For this review, take the finished solid that the model builds, in its own axes (mm). A direction names the side the tool comes from. Coordinates: 2 decimals unless noted, no trailing zeros. Order: outer loops, then holes, each group sorted by start corner. A loop starts at its lowest first (then second) coordinate and runs counter-clockwise, first axis right, second up. Notation, with made-up numbers: (29.5, 30) - (39.5, 30) arc R25 ccw to (39.5, 52) - close; hole circle Ø3 at (80.25, 0.5). An arc over 180 degrees is marked (long way). One line per item, written item: value. Start each with the question number.
(1) For faces 1 (the flat face through (238, 0, -1)), 2 (the flat face through (-3, 5, -50)), list the 3-axis set-ups (+Z, -Z, +X, -X, +Y, -Y) from which the entire face can be reached by the end or side of a thin tool; tool diameter is ignored.
(2) Clearance check with flat-ended pins moving along their axes: pin 1 (11 mm diameter, centred on x = 81.5, y = 6.5, fed in from -Z); pin 2 (5 mm diameter, centred on x = -92.5, z = -55.5, fed in from +Y). State where each tip first meets the part, or that it passes through.
(3) Consider section B-B on y = 4.25. Write out the cut boundary in (x, z), then the cut area to 3 significant figures.
(4) To check wall thickness, follow line 1 along Z through (x, y) = (-135, 6.5); line 2 along Y through (x, z) = (-32, -53.5). State the ranges of each line that lie inside material, in increasing order.
(5) Consider section A-A on x = -72.5. Write out the cut boundary in (y, z), then the cut area to 3 significant figures.
```python
from build123d import *

# Parameters (mm, degrees)
F0_W     = 476
F0_H     = 10
F1_DEPTH = 10
F0_H_2   = 110
F2_DEPTH = 10


with BuildPart() as f1:
    # F0 (on Front) → F1 (new body)
    with BuildSketch(Plane.XZ):
        with Locations((0, -55)):
            Rectangle(F0_W, F0_H)
    extrude(amount=F1_DEPTH)

    # F0 (on Front) → F2 (join, symmetric)
    with BuildSketch(Plane.XZ):
        with Locations((0, 5)):
            Rectangle(F0_W, F0_H_2)
    extrude(amount=F2_DEPTH, both=True)


solid = f1.part
```
Geometry check:
1. face 1: +Z, -Z, +X, +Y, -Y
1. face 2: -Z, +X, -X, +Y
2. pin 1: stops at z = -50
2. pin 2: stops at y = 0
3. outline: (-238, -50) - (238, -50) - (238, 60) - (-238, 60) - close
3. area: 52,400 mm^2
4. line 1: z = -50 to 60
4. line 2: y = -10 to 0
5. outline: (-10, -60) - (0, -60) - (0, -50) - (10, -50) - (10, 60) - (-10, 60) - close
5. area: 2,300 mm^2
